Design review of the part built by this model. Coordinates are the model's own, in mm. A direction names the side the tool comes from. Round coordinates to 2 decimals unless told otherwise and drop trailing zeros. Order: outer loops, then holes, each group sorted by start corner. A loop starts at its lowest first (then second) coordinate and runs counter-clockwise, first axis right, second up. Notation, with made-up numbers: (-21.75, -20.5) - (1.25, -20.5) arc R14 cw to (1.25, -5.5) - close; hole circle Ø9 at (84.5, 74). An arc over 180 degrees is marked (long way). Use CSV: the item, a comma, the result in double quotes.
from build123d import *

# Parameters (mm, degrees)
F0_R     = 17.5
F0_R_2   = 5
F1_DEPTH = 15
F2_R     = 17.5
F2_R_2   = 11
F3_DEPTH = 7
F6_R     = 17.5
F6_R_2   = 15.5
F7_DEPTH = 2


with BuildPart() as f1:
    # F0 (on Top) → F1 (new body)
    with BuildSketch(Plane.XY):
        Circle(F0_R)
        Circle(F0_R_2, mode=Mode.SUBTRACT)
    extrude(amount=F1_DEPTH)

    # F2 (on face) → F3 (join)
    with BuildSketch(Plane.XY.offset(15)):
        Circle(F2_R)
        Circle(F2_R_2, mode=Mode.SUBTRACT)
    extrude(amount=F3_DEPTH)

    # F4: F1 across plane


with BuildPart() as f1_1:
    add(f1.part)
    add(f1.part.mirror(Plane.XY))

    # F6 (on offset) → F7 (cut)
    with BuildSketch(Plane.XY.offset(15)):
        Circle(F6_R)
        Circle(F6_R_2, mode=Mode.SUBTRACT)
    extrude(amount=-F7_DEPTH, mode=Mode.SUBTRACT)


solid = f1_1.part
1) Insertion check: pin 1 Ø20 at (x, y) = (0, 0) entering from +Z; pin 2 Ø4 at (x, z) = (-2.5, 10) entering from +Y; pin 3 Ø1.5 at (y, z) = (-5, -8) entering from -X. Each pin has a flat end and moves straight along its axis. Give the tip position at first contact, or say it passes through.
Data:
pin 1,"stops at z = 15"
pin 2,"stops at y = 17.49"
pin 3,"stops at x = -16.98"
2) For faces 4 (the face through (-2.38, -10.74, 18.45)), 5 (the face through (-7, -14, 13)), 6 (the face through (8, 8, 22)), 7 (the face through (2, -5, -15)), 8 (the face through (-13.887, -10.648, -4.255)), list the 3-axis set-ups (+Z, -Z, +X, -X, +Y, -Y) from which the entire face can be reached by the end or side of a thin tool; tool diameter is ignored.
Data:
face 4,"+Z"
face 5,"none"
face 6,"+Z, +X, -X, +Y, -Y"
face 7,"-Z"
face 8,"+Z, -Z"
3) We need section C-C (z = 3). Give the boundary of the cut face in (x, y), then the cut area to 3 significant figures.
Data:
outline,"circle Ø35 at (0, 0); hole circle Ø10 at (0, 0)"
area,"884 mm2"
4) We need section A-A (x = 0). Give the boundary of the cut face in (y, z), then the cut area to 3 significant figures.
Data:
outline,"(-17.5, -22) - (-11, -22) - (-11, -15) - (-5, -15) - (-5, 15) - (-11, 15) - (-11, 22) - (-17.5, 22) - (-17.5, 15) - (-15.5, 15) - (-15.5, 13) - (-17.5, 13) - close; (5, -15) - (11, -15) - (11, -22) - (17.5, -22) - (17.5, 13) - (15.5, 13) - (15.5, 15) - (17.5, 15) - (17.5, 22) - (11, 22) - (11, 15) - (5, 15) - close"
area,"924 mm2"
5) The part is to be moulded in two halves that separate along Y. For faces 1 (the face through (-2.38, -10.74, -18.45)), 2 (the face through (-2.018, 15.368, 14.014)), 3 (the face through (-7, -14, 15)), say which applies: +Y half, -Y half, draft (parallel to the pull), parting line (faces both ways), or undercut.
Data:
face 1,"undercut"
face 2,"parting line"
face 3,"draft"
6) We need section D-D (x = 14.5). Give the boundary of the cut face in (y, z), then the cut area to 3 significant figures.
Data:
outline,"(-9.8, -22) - (9.8, -22) - (9.8, 13) - (5.48, 13) - (5.48, 15) - (9.8, 15) - (9.8, 22) - (-9.8, 22) - (-9.8, 15) - (-5.48, 15) - (-5.48, 13) - (-9.8, 13) - close"
area,"845 mm2"
7) To check wall thickness, follow L1, parallel to Y at x = 0, z = 17; L2, parallel to Y at x = 0, z = -8; L3, parallel to Z at x = 5, y = 7. State the ranges of each line that lie inside material, in increasing order. Write a range as from..to.
Data:
L1,"y = -17.5..-11, 11..17.5"
L2,"y = -17.5..-5, 5..17.5"
L3,"z = -15..15"
